Work out the finished part from the listing and answer in its coordinate system (mm). Face numbers are marked on the shaded views. A direction names the side the tool comes from. Round coordinates to 2 decimals unless told otherwise and drop trailing zeros. Loops run counter-clockwise (first coordinate to the right, second up) from the corner with the lowest first, then second, coordinate; pieces in that order, holes last.
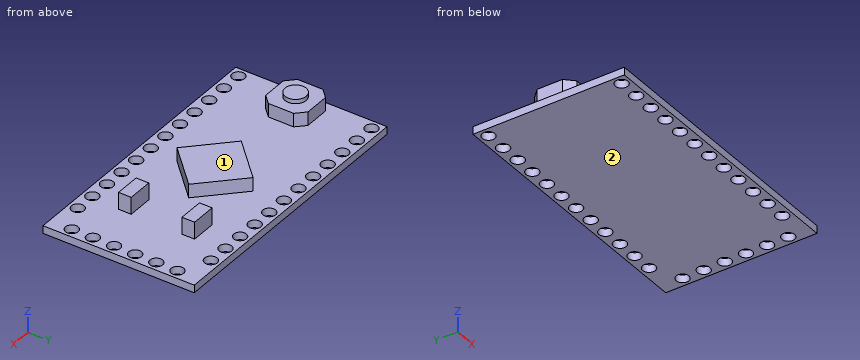
```python
from build123d import *

# Parameters (mm, degrees)
F0_W      = 33
F0_H      = 17.9
F1_DEPTH  = 0.9
F3_DEPTH  = 1.6
F5_DEPTH  = 1.6
F6_R      = 1.25
F7_DEPTH  = 0.5
F8_R      = 0.75
F9_DEPTH  = 25
F10_W     = 3
F10_H     = 1.5
F11_DEPTH = 2


with BuildPart() as f1:
    # F0 (on Top) → F1 (new body)
    with BuildSketch(Plane.XY):
        Rectangle(F0_W, F0_H)
    extrude(amount=F1_DEPTH)

    # F2 (on face) → F3 (join)
    with BuildSketch(Plane.XY.offset(0.9)):
        Polygon((4.5, 0), (0, 4.5), (-4.5, 0), (0, -4.5), align=None)
    extrude(amount=F3_DEPTH)

    # F4 (on face) → F5 (join)
    with BuildSketch(Plane.XY.offset(0.9)):
        Polygon((-12.3, 2.5), (-15.3, 2.5), (-16.3, 1.5), (-16.3, -1.5), (-15.3, -2.5), (-12.3, -2.5), (-11.3, -1.5), (-11.3, 1.5), align=None)
    extrude(amount=F5_DEPTH)

    # F6 (on face) → F7 (join)
    with BuildSketch(Plane.XY.offset(2.5)):
        with Locations((-13.8, 0)):
            Circle(F6_R)
    extrude(amount=F7_DEPTH)

    # F8 (on face) → F9 (cut)
    with BuildSketch(Plane.XY.offset(0.9)):
        with Locations((-15.4, 7.875409)):
            Circle(F8_R)
        with Locations((-12.9, 7.875409)):
            Circle(F8_R)
        with Locations((-10.4, 7.875409)):
            Circle(F8_R)
        with Locations((-7.9, 7.875409)):
            Circle(F8_R)
        with Locations((-5.4, 7.875409)):
            Circle(F8_R)
        with Locations((-2.9, 7.875409)):
            Circle(F8_R)
        with Locations((-0.4, 7.875409)):
            Circle(F8_R)
        with Locations((2.1, 7.875409)):
            Circle(F8_R)
        with Locations((4.6, 7.875409)):
            Circle(F8_R)
        with Locations((7.1, 7.875409)):
            Circle(F8_R)
        with Locations((9.6, 7.875409)):
            Circle(F8_R)
        with Locations((12.1, 7.875409)):
            Circle(F8_R)
        with Locations((-12.9, -7.875409)):
            Circle(F8_R)
        with Locations((-5.4, -7.875409)):
            Circle(F8_R)
        with Locations((-15.4, -7.875409)):
            Circle(F8_R)
        with Locations((-10.4, -7.875409)):
            Circle(F8_R)
        with Locations((-7.9, -7.875409)):
            Circle(F8_R)
        with Locations((12.1, -7.875409)):
            Circle(F8_R)
        with Locations((-2.9, -7.875409)):
            Circle(F8_R)
        with Locations((-0.4, -7.875409)):
            Circle(F8_R)
        with Locations((2.1, -7.875409)):
            Circle(F8_R)
        with Locations((4.6, -7.875409)):
            Circle(F8_R)
        with Locations((7.1, -7.875409)):
            Circle(F8_R)
        with Locations((9.6, -7.875409)):
            Circle(F8_R)
        with Locations((15.4, 6.2)):
            Circle(F8_R)
        with Locations((15.401431, 3.7)):
            Circle(F8_R)
        with Locations((15.402862, 1.200001)):
            Circle(F8_R)
        with Locations((15.404293, -1.299999)):
            Circle(F8_R)
        with Locations((15.405724, -3.799998)):
            Circle(F8_R)
        with Locations((15.407155, -6.299998)):
            Circle(F8_R)
    extrude(amount=-F9_DEPTH, mode=Mode.SUBTRACT)

    # F10 (on face) → F11 (join)
    with BuildSketch(Plane.XY.offset(0.9)):
        with Locations((8.5, 3.75)):
            Rectangle(F10_W, F10_H)
        with Locations((8.5, -3.75)):
            Rectangle(F10_W, F10_H)
    extrude(amount=F11_DEPTH)


solid = f1.part
```
1. Find section B-B (z = 1.4). Write down the section's boundary in (x, y), then the cut area to 3 significant figures.
Answer key:
outline: (-16.3, -1.5) - (-15.3, -2.5) - (-12.3, -2.5) - (-11.3, -1.5) - (-11.3, 1.5) - (-12.3, 2.5) - (-15.3, 2.5) - (-16.3, 1.5) - close; (-4.5, 0) - (0, -4.5) - (4.5, 0) - (0, 4.5) - close; (7, -4.5) - (10, -4.5) - (10, -3) - (7, -3) - close; (7, 3) - (10, 3) - (10, 4.5) - (7, 4.5) - close
area: 72.5 mm2
2. Consider probe 1 along Y at (x, z) = (-12.9, 0.45); probe 2 along X at (y, z) = (-1.25, 0.8); probe 3 along Z at (x, y) = (7, -6.25). Determine where each line is inside the solid, lowest interval first.
Answer key:
probe 1: y = -8.95 to -8.63, -7.13 to 7.13, 8.63 to 8.95
probe 2: x = -16.5 to 14.66, 16.15 to 16.5
probe 3: z = 0 to 0.9
3. Find section D-D (y = 6.2). Write down the section's boundary in (x, z).
Answer key:
outline: (-16.5, 0) - (14.65, 0) - (14.65, 0.9) - (-16.5, 0.9) - close; (16.15, 0) - (16.5, 0) - (16.5, 0.9) - (16.15, 0.9) - close
4. Given pin 1 (1.7 mm diameter, centred on x = 9.6, y = -7.88, fed in from +Z); pin 2 (5 mm diameter, centred on x = -1.5, y = 4.5, fed in from +Z); pin 3 (1.5 mm diameter, centred on x = -11, y = 3.5, fed in from -Z); pin 4 (0.8 mm diameter, centred on y = 4, z = 2.5, fed in from -X), each flat-ended and moving along its own axis, determine where each tip first touches the part or whether it passes through.
Answer key:
pin 1: stops at z = 0.9
pin 2: stops at z = 2.5
pin 3: stops at z = 0
pin 4: stops at x = -0.9
5. Which of the six approach directions +Z, -Z, +X, -X, +Y, -Y give full straight-line access (tool end or side, diameter ignored) to the marked faces 1 and 2?
Answer key:
face 1: +Z, +Y, -Y
face 2: -Z, +X, -X, +Y, -Y
6. Find section A-A (y = 3.7). Write down the section's boundary in (x, z), then the cut area to 3 significant figures.
Answer key:
outline: (-16.5, 0) - (14.65, 0) - (14.65, 0.9) - (10, 0.9) - (10, 2.9) - (7, 2.9) - (7, 0.9) - (0.8, 0.9) - (0.8, 2.5) - (-0.8, 2.5) - (-0.8, 0.9) - (-16.5, 0.9) - close; (16.15, 0) - (16.5, 0) - (16.5, 0.9) - (16.15, 0.9) - close
area: 36.9 mm2
7. Find section C-C (x = 9.6). Write down the section's boundary in (y, z).
Answer key:
outline: (-8.95, 0) - (-8.63, 0) - (-8.63, 0.9) - (-8.95, 0.9) - close; (-7.13, 0) - (7.13, 0) - (7.13, 0.9) - (4.5, 0.9) - (4.5, 2.9) - (3, 2.9) - (3, 0.9) - (-3, 0.9) - (-3, 2.9) - (-4.5, 2.9) - (-4.5, 0.9) - (-7.13, 0.9) - close; (8.63, 0) - (8.95, 0) - (8.95, 0.9) - (8.63, 0.9) - close
